Answer from the drawing. Dimensions are ordinates in mm from the lowest x, y and z of the part. Coordinates: 2 decimals unless noted, no trailing zeros. Write each loop counter-clockwise with the first axis right and the second up, starting at its lowest first coordinate (ties: lowest second). Pieces come first, ordered by that corner, then holes.
(1) The part is cut by section D-D, the plane z = 19.5. Determine the outline of the cut face in (x, y), and give its area (3 significant figures).
(2) Determine the mould class of the marked faces 1, 2 and 3 for opening direction X: pulls with the +X half, pulls with the -X half, needs draft (parallel to the pull), parting line crosses it, or undercut.
(3) The part is cut by section A-A, the plane z = 15.5. Determine the outline of the cut face in (x, y), and give its area (3 significant figures).
(4) The part is cut by section C-C, the plane y = 2.95. Determine the outline of the cut face in (x, z), and give its area (3 significant figures).
(5) Straight lines are drawn through the part: line 1 along Z through (x, y) = (18.5, 0.5); line 2 along X through (y, z) = (2.45, 28.5); line 3 along Z through (x, y) = (17.5, 0.45). For each, find the intervals that lie inside material, in ascending order.
(6) Given pin 1 (1 mm diameter, centred on y = 3.5, z = 21, fed in from +X); pin 2 (1.5 mm diameter, centred on x = 20, y = 2.5, fed in from +Z); pin 3 (1.5 mm diameter, centred on x = 7, y = 1.5, fed in from -Z), each flat-ended and moving along its own axis, determine where each tip first touches the part or whether it passes through.
(7) The part is cut by section B-B, the plane x = 28.5. Determine the outline of the cut face in (y, z).
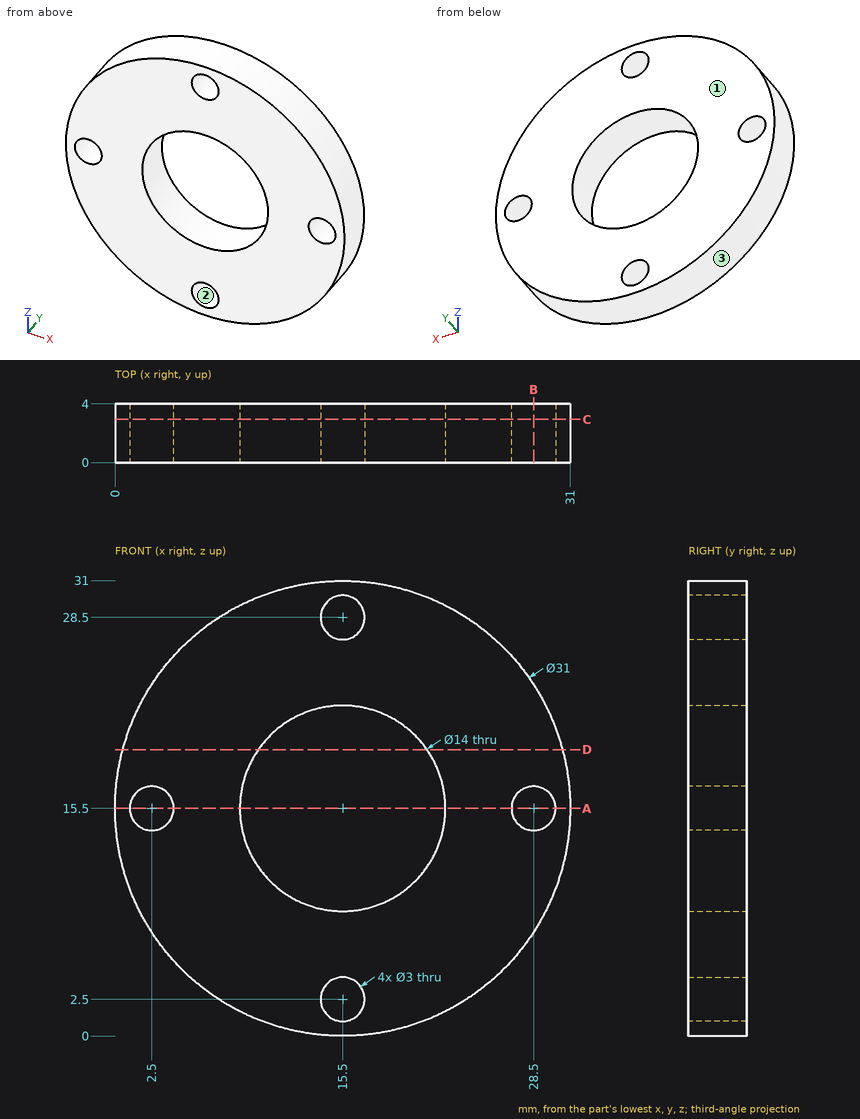
Computed:
1. outline: (0.53, 0) - (9.76, 0) - (9.76, 4) - (0.53, 4) - close; (21.24, 0) - (30.47, 0) - (30.47, 4) - (21.24, 4) - close
1. area: 73.8 mm2
2. face 1: needs draft
2. face 2: undercut
2. face 3: parting line crosses it
3. outline: (0, 0) - (1, 0) - (1, 4) - (0, 4) - close; (4, 0) - (8.5, 0) - (8.5, 4) - (4, 4) - close; (22.5, 0) - (27, 0) - (27, 4) - (22.5, 4) - close; (30, 0) - (31, 0) - (31, 4) - (30, 4) - close
3. area: 44.0 mm2
4. outline: circle Ø31 at (15.5, 15.5); hole circle Ø3 at (2.5, 15.5); hole circle Ø14 at (15.5, 15.5); hole circle Ø3 at (15.5, 2.5); hole circle Ø3 at (15.5, 28.5); hole circle Ø3 at (28.5, 15.5)
4. area: 573 mm2
5. line 1: z = 0.29 to 9.18, 21.82 to 30.71
5. line 2: x = 7.06 to 14, 17 to 23.94
5. line 3: z = 0.13 to 8.79, 22.21 to 30.87
6. pin 1: stops at x = 30.17
6. pin 2: stops at z = 30.54
6. pin 3: stops at z = 2.08
7. outline: (0, 7.06) - (4, 7.06) - (4, 14) - (0, 14) - close; (0, 17) - (4, 17) - (4, 23.94) - (0, 23.94) - close
